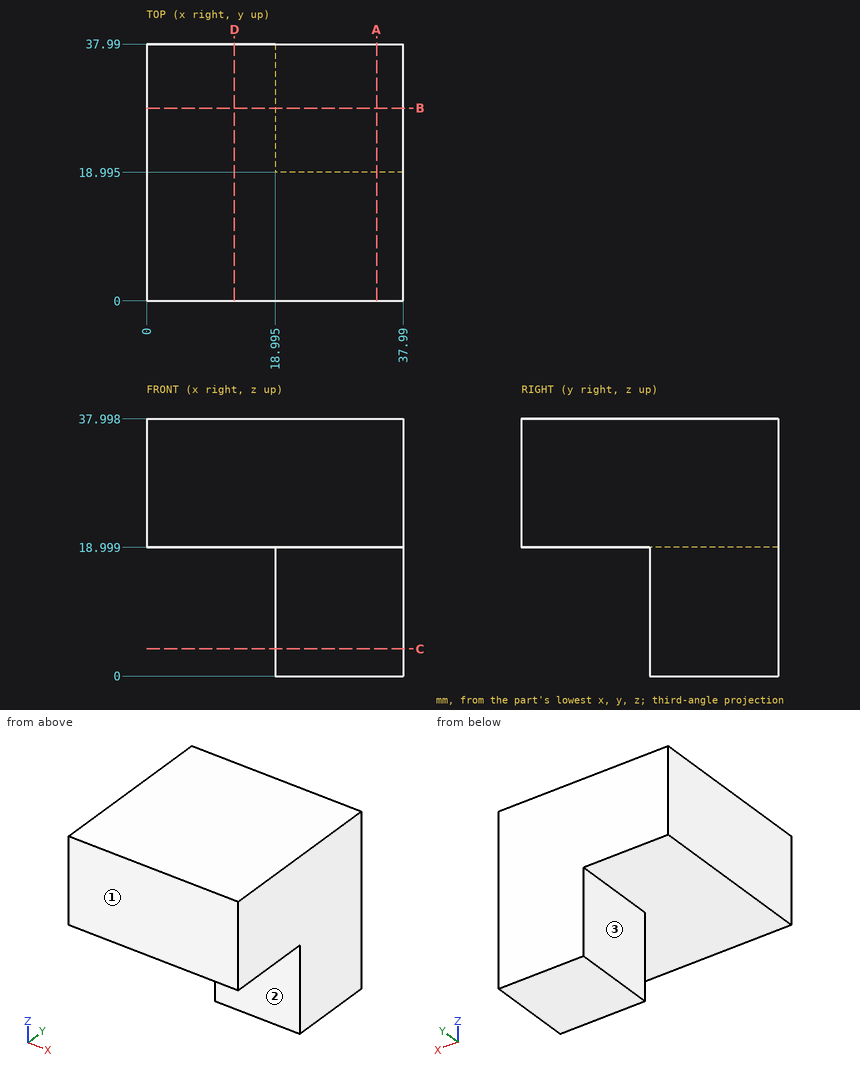
Geometry: see drawing. Coordinates: mm, zero at the bounding-box minimum. A direction names the side the tool comes from. Give positions to 0.01 mm unless a question says otherwise; leave off trailing zeros. Loops run counter-clockwise (first coordinate to the right, second up) from the corner with the lowest first, then second, coordinate; pieces in that order, holes last. Notation, with made-up numbers: (-1.5, 32.5) -> (53.5, 32.5) arc R19 ccw to (53.5, 53.5) -> close; hole circle Ø5 at (80.5, -10). An arc over 180 degrees is marked (long way). Use CSV: the item, a comma, the result in double quotes.
(1) Cut plane C-C (z = 4). Output: boundary loops of the cut face in (x, y) (1 decimal).
From the geometry:
outline,"(19, 19) -> (38, 19) -> (38, 38) -> (19, 38) -> close"
(2) Cut plane D-D (x = 13). Output: boundary loops of the cut face in (y, z).
From the geometry:
outline,"(0, 19) -> (37.99, 19) -> (37.99, 38) -> (0, 38) -> close"
(3) Access query for the marked faces 1, 2 and 3. Directions: +Z, -Z, +X, -X, +Y, -Y. A direction counts if a zero-diameter tool reaches every point of the face in a straight line with its end or side. Return the directions, or none.
From the geometry:
face 1,"+Z, -Z, +X, -X, -Y"
face 2,"-Z, +X, -X, -Y"
face 3,"-Z, -X, +Y, -Y"
(4) Ray query, line 1 along Y through (x, z) = (24, 3) (1 decimal). Return the intervals inside material, ascending. Write a range as [from, to].
From the geometry:
line 1,"[19, 38]"
(5) Cut plane A-A (x = 34). Output: boundary loops of the cut face in (y, z) (1 decimal), plus the area to 3 significant figures.
From the geometry:
outline,"(0, 19) -> (19, 19) -> (19, 0) -> (38, 0) -> (38, 38) -> (0, 38) -> close"
area,"1,080 mm^2"
(6) First-contact query: P1, Ø8, axis at y = 14.5, z = 10, coming from the +X side; P2, Ø5.5, axis at y = 27.5, z = 6, coming from the -X side (1 decimal); P3, Ø5.5, axis at x = 31.5, z = 9.5, coming from the -Y side (1 decimal). Flat tips, straight axial feed; report the tip coordinate or a pass-through.
From the geometry:
P1,"through"
P2,"x = 19"
P3,"y = 19"
